from build123d import *

# Parameters (mm, degrees)
SKETCH_1_W          = 40
SKETCH_1_H          = 14
EXTRUDE_1_DEPTH     = 60
SKETCH_6_W          = 36
SKETCH_6_H          = 10
CUT_EXTRUDE_2_DEPTH = 55
SKETCH_7_W          = 40
SKETCH_7_H          = 10
CUT_EXTRUDE_3_DEPTH = 7
SKETCH_15_OUTSIDE_W = 56.692
SKETCH_15_OUTSIDE_H = 30.692
CUT_EXTRUDE_5_DEPTH = 61


with BuildPart() as part:
    # 草图1 → 凸台-拉伸1 (new body)
    with BuildSketch(Plane(origin=(0, 0, 0), x_dir=(1, 0, 0), z_dir=(0, 1, 0))):
        with Locations((20, 7)):
            Rectangle(SKETCH_1_W, SKETCH_1_H)
    extrude(amount=EXTRUDE_1_DEPTH)

    # 草图6 → 切除-拉伸2 (cut)
    with BuildSketch(Plane(origin=(0, 60, 0), x_dir=(1, 0, 0), z_dir=(0, 1, 0))):
        with Locations((20, 7)):
            Rectangle(SKETCH_6_W, SKETCH_6_H)
    extrude(amount=-CUT_EXTRUDE_2_DEPTH, mode=Mode.SUBTRACT)

    # 草图7 → 切除-拉伸3 (cut)
    with BuildSketch(Plane.XY):
        with Locations((20, 55)):
            Rectangle(SKETCH_7_W, SKETCH_7_H)
    extrude(amount=-CUT_EXTRUDE_3_DEPTH, mode=Mode.SUBTRACT)

    # 草图15 outside → 切除-拉伸5 (cut, through all)
    with BuildSketch(Plane.XZ):
        with Locations((20, -7)):
            Rectangle(SKETCH_15_OUTSIDE_W, SKETCH_15_OUTSIDE_H)
        with BuildLine():
            Line((2, -14), (38, -14))
            ThreePointArc((38, -14), (39.414213562, -13.414213562), (40, -12))
            Line((40, -12), (40, -2))
            ThreePointArc((40, -2), (39.414213562, -0.585786438), (38, 0))
            Line((38, 0), (2, 0))
            ThreePointArc((2, 0), (0.585786438, -0.585786438), (0, -2))
            Line((0, -2), (0, -12))
            ThreePointArc((0, -12), (0.585786438, -13.414213562), (2, -14))
        make_face(mode=Mode.SUBTRACT)
    extrude(amount=-CUT_EXTRUDE_5_DEPTH, mode=Mode.SUBTRACT)


solid = part.part
Design review of the part built by this model. Coordinates are the model's own, in mm. A direction names the side the tool comes from. Coordinates: 2 decimals unless noted, no trailing zeros. Order: outer loops, then holes, each group sorted by start corner. A loop starts at its lowest first (then second) coordinate and runs counter-clockwise, first axis right, second up. Notation, with made-up numbers: M 25,32.5 L 59,32.5 A10 ccw 59,49.5 Z; hole C 52,-36.5 d1. An arc over 180 degrees is marked long. Use a Markdown table: item, result.
(1) For P1, Ø5.5, axis at x = 18.5, z = -4.5, coming from the +Y side; P2, Ø1, axis at x = 39, y = 54, coming from the +Z side; P3, Ø4, axis at x = 5.5, z = -5, coming from the +Y side, all flat-tipped, find the tip position at first contact; note any pin that passes through.
Worked answers:
| item | result |
|---|---|
| P1 | stops at y = 50 |
| P2 | stops at z = -7 |
| P3 | stops at y = 5 |
(2) Wall thickness on probe 1 along X at (y, z) = (51.5, -7.75); probe 2 along Z at (x, y) = (18.5, 12.5); probe 3 along Y at (x, z) = (30, -10.5): over which ranges is each line inside the solid? List them lowest first.
Worked answers:
| item | result |
|---|---|
| probe 1 | x = 0 to 2, 38 to 40 |
| probe 2 | z = -14 to -12, -2 to 0 |
| probe 3 | y = 0 to 5 |
(3) Draft analysis for pull direction Z (two halves, no side actions). For faces 1 (the cylindrical face through (0.6, 24.65, -0.57)), 2 (the cylindrical face through (39.4, 29.58, -13.43)), 3 (the flat face through (38, 33, -7)), 4 (the flat face through (20, 28, -2)), state which applies: released by +Z, released by -Z, zero draft, split by the parting line, or undercut.
Worked answers:
| item | result |
|---|---|
| face 1 | released by +Z |
| face 2 | released by -Z |
| face 3 | undercut |
| face 4 | undercut |
(4) Add section A-A (y = 16.5). Give the boundary of the cut face in (x, z), then the cut area to 3 significant figures.
Worked answers:
| item | result |
|---|---|
| outline | M 0,-12 A2 ccw 2,-14 L 38,-14 A2 ccw 40,-12 L 40,-2 A2 ccw 38,0 L 2,0 A2 ccw 0,-2 Z; hole M 2,-12 L 38,-12 L 38,-2 L 2,-2 Z |
| area | 197 mm2 |
(5) For faces 5 (the flat face through (39, 55, -7)), 6 (the flat face through (20, 5, -7)), 7 (the flat face through (40, 30, -7)), list the 3-axis set-ups (+Z, -Z, +X, -X, +Y, -Y) from which the entire face can be reached by the end or side of a thin tool; tool diameter is ignored.
Worked answers:
| item | result |
|---|---|
| face 5 | +Z, +X, -X, +Y |
| face 6 | +Y |
| face 7 | +Z, -Z, +X, +Y, -Y |
(6) Add section C-C (z = -4.75). Give the boundary of the cut face in (x, y).
Worked answers:
| item | result |
|---|---|
| outline | M 0,0 L 40,0 L 40,50 L 38,50 L 38,5 L 2,5 L 2,50 L 0,50 Z |
(7) Add section D-D (y = 51.5). Give the boundary of the cut face in (x, z).
Worked answers:
| item | result |
|---|---|
| outline | M 0,-12 A2 ccw 2,-14 L 38,-14 A2 ccw 40,-12 L 40,-7 L 38,-7 L 38,-12 L 2,-12 L 2,-7 L 0,-7 Z |
(8) Add section B-B (x = 4.5). Give the boundary of the cut face in (y, z), then the cut area to 3 significant figures.
Worked answers:
| item | result |
|---|---|
| outline | M 0,-14 L 60,-14 L 60,-12 L 5,-12 L 5,-2 L 50,-2 L 50,0 L 0,0 Z |
| area | 270 mm2 |
